Answer from the drawing. Dimensions are ordinates in mm from the lowest x, y and z of the part. Round coordinates to 2 decimals unless told otherwise and drop trailing zeros. Write each loop counter-clockwise with the first axis right and the second up, starting at its lowest first coordinate (ties: lowest second). Pieces come first, ordered by that corner, then holes. Notation, with made-up numbers: M 26,-7.5 L 32,-7.5 A30 cw 32,26.5 Z; hole C 25,42 d6. An arc over 180 degrees is marked long. One line per item, written item: value. Start each with the question number.
(1) Section A-A (z = 18.5) is taken. Determine the outline of the cut face in (x, y).
(2) Section C-C (y = 18.75) is taken. Determine the outline of the cut face in (x, z), plus the area to 3 significant figures.
(3) Given P1, Ø6, axis at x = 15.5, z = 17, coming from the +Y side; P2, Ø8, axis at y = 12.5, z = 11, coming from the +X side; P3, Ø4.5, axis at y = 3, z = 6.5, coming from the -X side (3 decimals); P4, Ø5, axis at x = 44.5, y = 16, coming from the +Z side, each flat-ended and moving along its own axis, determine where each tip first touches the part or whether it passes through.
(4) Section D-D (x = 26) is taken. Determine the outline of the cut face in (y, z), plus the area to 3 significant figures.
(5) Consider probe 1 along Z at (x, y) = (49.27, 25); probe 2 along X at (y, z) = (28.25, 26.15); probe 3 along X at (y, z) = (3.75, 6.75). Determine where each line is inside the solid, lowest interval first.
(6) For a pull along X with two mould halves and no side action, classify the marked faces 1, 2 and 3 as released by +X, released by -X, zero draft, split by the parting line, or undercut.
(7) Section B-B (y = 27.25) is taken. Determine the outline of the cut face in (x, z), plus the area to 3 significant figures.
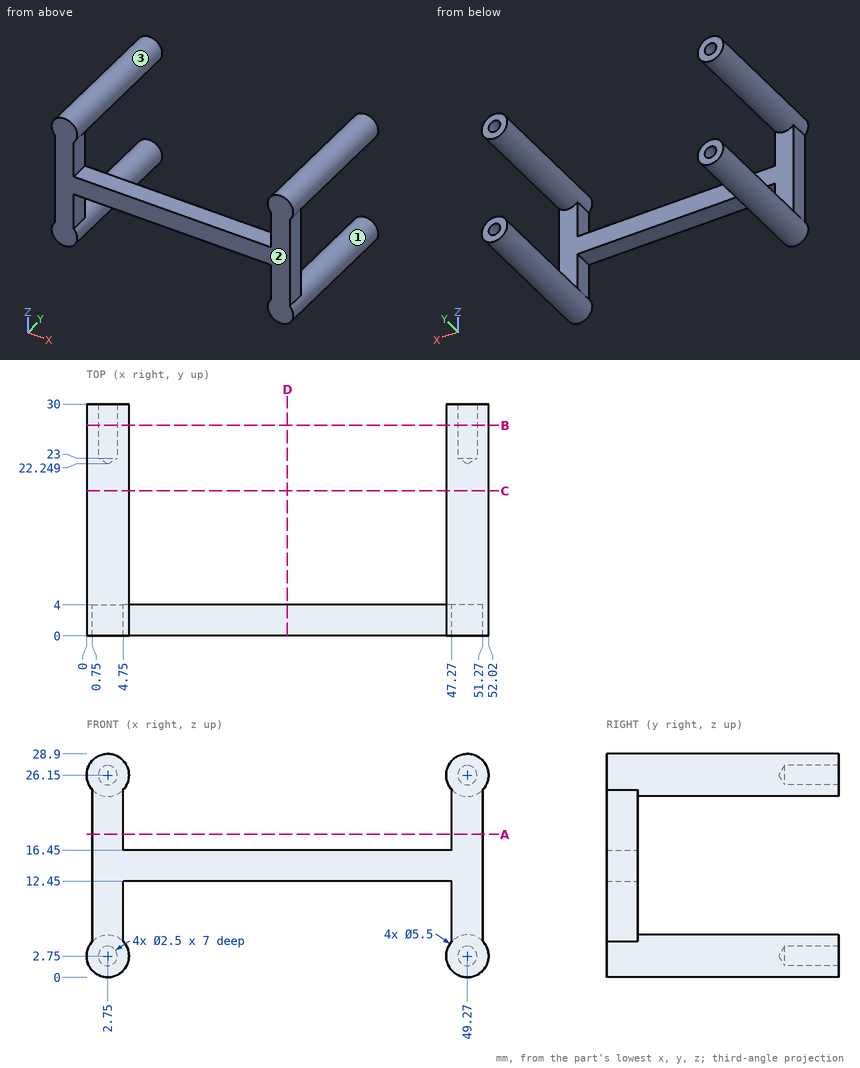
Recorded:
1. outline: M 0.75,0 L 4.75,0 L 4.75,4 L 0.75,4 Z; M 47.27,0 L 51.27,0 L 51.27,4 L 47.27,4 Z
2. outline: C 2.75,2.75 d5.5; C 2.75,26.15 d5.5; C 49.27,2.75 d5.5; C 49.27,26.15 d5.5
2. area: 95.0 mm2
3. P1: stops at y = 4
3. P2: passes through
3. P3: stops at x = 0.445
3. P4: stops at z = 27.7
4. outline: M 0,12.45 L 4,12.45 L 4,16.45 L 0,16.45 Z
4. area: 16.0 mm2
5. probe 1: z = 0 to 1.5, 4 to 5.5, 23.4 to 24.9, 27.4 to 28.9
5. probe 2: x = 0 to 1.5, 4 to 5.5, 46.52 to 48.02, 50.52 to 52.02
5. probe 3: x = 0.75 to 4.75, 47.27 to 51.27
6. face 1: undercut
6. face 2: zero draft
6. face 3: undercut
7. outline: C 2.75,2.75 d5.5; C 2.75,26.15 d5.5; C 49.27,2.75 d5.5; C 49.27,26.15 d5.5; hole C 2.75,2.75 d2.5; hole C 2.75,26.15 d2.5; hole C 49.27,2.75 d2.5; hole C 49.27,26.15 d2.5
7. area: 75.4 mm2
